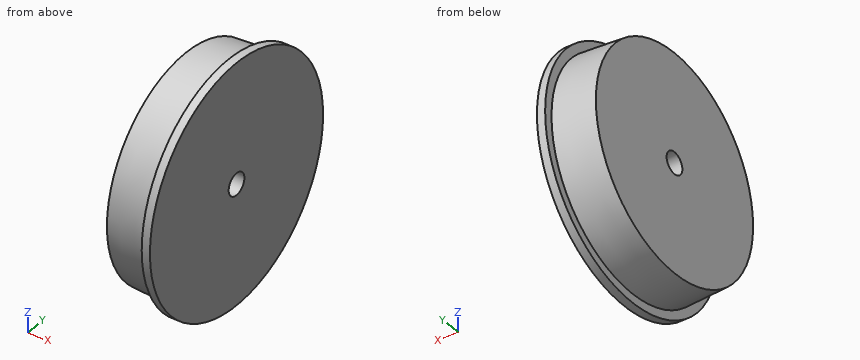
from build123d import *

# Parameters (mm, degrees)
SKETCH2_R           = 20
CUT_EXTRUDE1_DEPTH  = 299.977701101
SKETCH3_R           = 220.25163117
SKETCH3_R_2         = 20
BOSS_EXTRUDE1_DEPTH = 15


with BuildPart() as part:
    # Sketch1 → Revolve1 (revolve)
    with BuildSketch(Plane.XY):
        Polygon((0, 0), (-78, 0), (-78, 200), (0, 204.087806784), align=None)
    revolve(axis=Axis((0, 0, 0), (-1, 0, 0)))

    # Sketch2 → Cut-Extrude1 (cut, through all)
    with BuildSketch(Plane.ZY.offset(78)):
        with Locations(Location((0, 0, 0), (0, 0, 270))):
            Circle(SKETCH2_R)
    extrude(amount=-CUT_EXTRUDE1_DEPTH, mode=Mode.SUBTRACT)

    # Sketch3 → Boss-Extrude1 (add)
    with BuildSketch(Plane(origin=(0, 0, 0), x_dir=(0, 0, -1), z_dir=(1, 0, 0))):
        with Locations(Location((0, 0, 0), (0, 0, 90))):
            Circle(SKETCH3_R)
        with Locations(Location((0, 0, 0), (0, 0, 270))):
            Circle(SKETCH3_R_2, mode=Mode.SUBTRACT)
    extrude(amount=BOSS_EXTRUDE1_DEPTH)


solid = part.part
CAD build for the part. Positions are in the model's coordinates, mm. Round coordinates to 2 decimals unless told otherwise and drop trailing zeros. Loops run counter-clockwise (first coordinate to the right, second up) from the corner with the lowest first, then second, coordinate; pieces in that order, holes last.
(1) Drop flat-ended pins along their axis: pin 1 (1 mm diameter, centred on x = -6.5, y = 37, fed in from +Z); pin 2 (4 mm diameter, centred on x = -10.5, z = 90.5, fed in from -Y); pin 3 (4 mm diameter, centred on x = 5.5, y = 85, fed in from -Z). Give the stop position or say it passes through.
(2) Cut at A-A (z = 0). Give the cut face in (x, y), plus the area to 3 significant figures.
(3) Wall check: line 1 along Z through (x, y) = (-35, 0); line 2 along Y through (x, z) = (-30, 0); line 3 along Y through (x, z) = (-9.5, 0). Give the ranges that are in metal, low to high.
Findings below:
1. pin 1: stops at z = 200.45
1. pin 2: stops at y = -183.3
1. pin 3: stops at z = -204.01
2. outline: (-78, -200) - (0, -204.09) - (0, -220.25) - (15, -220.25) - (15, -20) - (-78, -20) - close; (-78, 20) - (15, 20) - (15, 220.25) - (0, 220.25) - (0, 204.09) - (-78, 200) - close
2. area: 34,400 mm2
3. line 1: z = -202.25 to -20, 20 to 202.25
3. line 2: y = -202.52 to -20, 20 to 202.52
3. line 3: y = -203.59 to -20, 20 to 203.59
